from build123d import *

# Parameters (mm, degrees)
SKETCH1_W           = 82.55
SKETCH1_H           = 69.85
BOSS_EXTRUDE1_DEPTH = 19.05
CUT_EXTRUDE2_START  = -19.05
SKETCH2_R           = 5.08
CUT_EXTRUDE2_DEPTH  = 38.1
CUT_EXTRUDE4_START  = -19.05
SKETCH3_R           = 5.08
CUT_EXTRUDE4_DEPTH  = 38.1
CUT_EXTRUDE6_START  = 19.05
SKETCH4_R           = 7.366
CUT_EXTRUDE6_DEPTH  = 12.7
CUT_EXTRUDE8_START  = 19.05
SKETCH5_R           = 12.7254
CUT_EXTRUDE8_DEPTH  = 2.8194
CUT_EXTRUDE10_START = 19.05
SKETCH6_R           = 7.366
CUT_EXTRUDE10_DEPTH = 12.7
CUT_EXTRUDE12_START = 19.05
SKETCH7_R           = 12.7254
CUT_EXTRUDE12_DEPTH = 2.8194


with BuildPart() as part:
    # Sketch1 → Boss-Extrude1 (new, symmetric)
    with BuildSketch(Plane(origin=(0, 0, 0), x_dir=(0, 1, 0), z_dir=(0, 0, 1))):
        Rectangle(SKETCH1_W, SKETCH1_H)
    extrude(amount=BOSS_EXTRUDE1_DEPTH, both=True)

    # Sketch2 → Cut-Extrude2 (cut)
    with BuildSketch(Plane(origin=(0, 0, 0), x_dir=(0, 1, 0), z_dir=(0, 0, 1)).offset(CUT_EXTRUDE2_START)):
        with Locations(Location((-30.226, -23.876, 0), (0, 0, 270))):
            Circle(SKETCH2_R)
    extrude(amount=CUT_EXTRUDE2_DEPTH, mode=Mode.SUBTRACT)

    # Sketch3 → Cut-Extrude4 (cut)
    with BuildSketch(Plane(origin=(0, 0, 0), x_dir=(0, 1, 0), z_dir=(0, 0, 1)).offset(CUT_EXTRUDE4_START)):
        with Locations(Location((30.226, -23.876, 0), (0, 0, 270))):
            Circle(SKETCH3_R)
        with Locations(Location((-30.226, 23.876, 0), (0, 0, 270))):
            Circle(SKETCH3_R)
        with Locations(Location((30.226, 23.876, 0), (0, 0, 270))):
            Circle(SKETCH3_R)
    extrude(amount=CUT_EXTRUDE4_DEPTH, mode=Mode.SUBTRACT)

    # Sketch4 → Cut-Extrude6 (cut)
    with BuildSketch(Plane(origin=(0, 0, 0), x_dir=(0, 1, 0), z_dir=(0, 0, 1)).offset(CUT_EXTRUDE6_START)):
        with Locations(Location((-17.526, 0, 0), (0, 0, 270))):
            Circle(SKETCH4_R)
    extrude(amount=-CUT_EXTRUDE6_DEPTH, mode=Mode.SUBTRACT)

    # Sketch5 → Cut-Extrude8 (cut)
    with BuildSketch(Plane(origin=(0, 0, 0), x_dir=(0, 1, 0), z_dir=(0, 0, 1)).offset(CUT_EXTRUDE8_START)):
        with Locations(Location((-17.526, 0, 0), (0, 0, 270))):
            Circle(SKETCH5_R)
    extrude(amount=-CUT_EXTRUDE8_DEPTH, mode=Mode.SUBTRACT)

    # Sketch6 → Cut-Extrude10 (cut)
    with BuildSketch(Plane(origin=(0, 0, 0), x_dir=(0, 1, 0), z_dir=(0, 0, 1)).offset(CUT_EXTRUDE10_START)):
        with Locations(Location((17.526, 0, 0), (0, 0, 270))):
            Circle(SKETCH6_R)
    extrude(amount=-CUT_EXTRUDE10_DEPTH, mode=Mode.SUBTRACT)

    # Sketch7 → Cut-Extrude12 (cut)
    with BuildSketch(Plane(origin=(0, 0, 0), x_dir=(0, 1, 0), z_dir=(0, 0, 1)).offset(CUT_EXTRUDE12_START)):
        with Locations(Location((17.526, 0, 0), (0, 0, 270))):
            Circle(SKETCH7_R)
    extrude(amount=-CUT_EXTRUDE12_DEPTH, mode=Mode.SUBTRACT)


solid = part.part
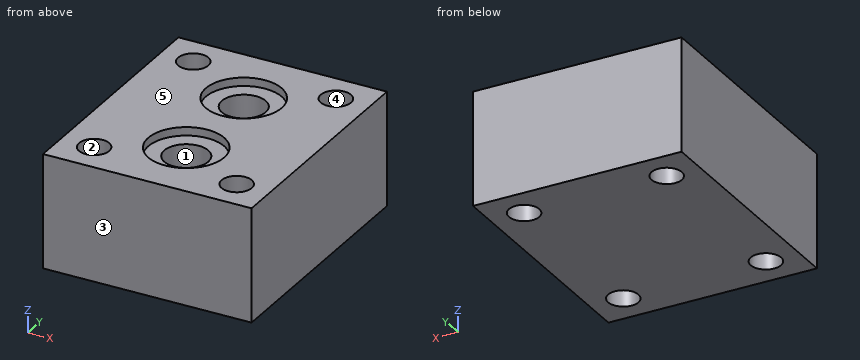
Input: part model. Units: mm. Frame: model coordinates. Face numbers are marked on the shaded views. A direction names the side the tool comes from. Round coordinates to 2 decimals unless told otherwise and drop trailing zeros. Loops run counter-clockwise (first coordinate to the right, second up) from the corner with the lowest first, then second, coordinate; pieces in that order, holes last. Notation, with made-up numbers: (14, 79.5) -> (56, 79.5) arc R27 ccw to (56, 110.5) -> close; hole circle Ø8 at (89.25, 87.5). An arc over 180 degrees is marked (long way). Answer as a JSON object with one key per item and string values. Group by question number.
1) Section query D-D on y = 22. Output: boundary loops of the cut face in (x, z) (3 decimals).
2) Section query A-A on x = 0. Output: boundary loops of the cut face in (y, z) (3 decimals), plus the area to 3 significant figures.
3) Ray query, L1, parallel to Y at x = 0, z = 17.8 (3 decimals); L2, parallel to Y at x = -26, z = -10.5 (3 decimals); L3, parallel to X at y = -18, z = 16 (3 decimals). Return the intervals inside material, ascending.
4) Section query B-B on z = 10. Output: boundary loops of the cut face in (x, y) (3 decimals).
5) Draft query along Y for the marked faces 3, 4 and 5. Return one class per face: +Y half, -Y half, draft (parallel to the pull), parting line (faces both ways), or undercut.
6) Reachability of the marked faces 1 and 2 from +Z, -Z, +X, -X, +Y, -Y: full face, straight path, thin tool, end or side. Return the list, or none.
7) Pin query (flat end, axial travel): pin 1 (8 mm diameter, centred on x = 3.5, y = 28, fed in from +Z); pin 2 (16 mm diameter, centred on x = -2.5, y = -18.5, fed in from +Z); pin 3 (9 mm diameter, centred on x = 0, y = 17.526, fed in from +Z). Return the tip coordinate at first contact, or that it passes through.
8) Section query C-C on x = 24. Output: boundary loops of the cut face in (y, z) (3 decimals).
Reply:
{
 "1": {"outline": "(-34.925, -19.05) -> (34.925, -19.05) -> (34.925, 19.05) -> (11.913, 19.05) -> (11.913, 16.231) -> (5.852, 16.231) -> (5.852, 6.35) -> (-5.852, 6.35) -> (-5.852, 16.231) -> (-11.913, 16.231) -> (-11.913, 19.05) -> (-34.925, 19.05) -> close"},
 "2": {"outline": "(-41.275, -19.05) -> (41.275, -19.05) -> (41.275, 19.05) -> (30.251, 19.05) -> (30.251, 16.231) -> (24.892, 16.231) -> (24.892, 6.35) -> (10.16, 6.35) -> (10.16, 16.231) -> (4.801, 16.231) -> (4.801, 19.05) -> (-4.801, 19.05) -> (-4.801, 16.231) -> (-10.16, 16.231) -> (-10.16, 6.35) -> (-24.892, 6.35) -> (-24.892, 16.231) -> (-30.251, 16.231) -> (-30.251, 19.05) -> (-41.275, 19.05) -> close", "area": "2,710 mm2"},
 "3": {"L1": "y = -41.275 to -30.251, -4.801 to 4.801, 30.251 to 41.275", "L2": "y = -41.275 to -34.841, -25.611 to 25.611, 34.841 to 41.275", "L3": "x = -34.925 to -7.351, 7.351 to 34.925"},
 "4": {"outline": "(-34.925, -41.275) -> (34.925, -41.275) -> (34.925, 41.275) -> (-34.925, 41.275) -> close; hole circle Ø10.16 at (-23.876, -30.226); hole circle Ø10.16 at (-23.876, 30.226); hole circle Ø14.732 at (0, -17.526); hole circle Ø14.732 at (0, 17.526); hole circle Ø10.16 at (23.876, -30.226); hole circle Ø10.16 at (23.876, 30.226)"},
 "5": {"face 3": "-Y half", "face 4": "undercut", "face 5": "draft"},
 "6": {"face 1": "+Z", "face 2": "+Z, -Z"},
 "7": {"pin 1": "stops at z = 19.05", "pin 2": "stops at z = 16.23", "pin 3": "stops at z = 6.35"},
 "8": {"outline": "(-41.275, -19.05) -> (-35.304, -19.05) -> (-35.304, 19.05) -> (-41.275, 19.05) -> close; (-25.148, -19.05) -> (25.148, -19.05) -> (25.148, 19.05) -> (-25.148, 19.05) -> close; (35.304, -19.05) -> (41.275, -19.05) -> (41.275, 19.05) -> (35.304, 19.05) -> close"}
}
